Read the model definition and answer for the solid it produces. Units are mm, in the model's axes. A direction names the side the tool comes from. Coordinates: 2 decimals unless noted, no trailing zeros. Write each loop counter-clockwise with the first axis right and the second up, starting at its lowest first coordinate (ties: lowest second). Pieces come first, ordered by that corner, then holes. Notation, with made-up numbers: (18.25, 11.5) -> (36.25, 11.5) arc R23 ccw to (36.25, 43.5) -> close; hole circle Ø5 at (10, 40). An arc over 180 degrees is marked (long way). Answer as a JSON object with one key per item and string values. Group by question number.
(1) Which of the six approach directions +Z, -Z, +X, -X, +Y, -Y give full straight-line access (tool end or side, diameter ignored) to faces 4 (the face through (2.66, 200.25, -67.4)), 5 (the face through (3, 2, -12.75)), 6 (the face through (6, 175, -100)), 7 (the face through (4.93, 68.93, -91.5))?
(2) Find section A-A (y = 168.5). Give the vertices of the cut face in (x, z).
(3) Find section B-B (y = 89.4). Give the vertices of the cut face in (x, z).
(4) For a pull along Z with two mould halves and no side action, classify faces 1 (the face through (8, 8, -67)), 2 (the face through (5.4, 3, -15)), 3 (the face through (4.93, 16.93, -126.5)) as +Z half, -Z half, draft (parallel to the pull), parting line (faces both ways), or undercut.
(5) Straight lines are drawn through the part: L1, parallel to Y at x = 3.3, z = -100; L2, parallel to Z at x = 5, y = 168.5; L3, parallel to Z at x = 4.35, y = 175. For each, find the intervals that lie inside material, in ascending order.
(6) A flat-ended cylindrical pin translates along its axis: P1, Ø1.6, axis at x = 5, y = 188.5, coming from the -Z side. Find the tip coordinate at first contact, or state that the pin passes through.
from build123d import *

# Parameters (mm, degrees)
SKETCH1_W                  = 135
SKETCH1_H                  = 210
BOSS_EXTRUDE1_DEPTH        = 10
SKETCH2_W                  = 45
SKETCH2_H                  = 60
CUT_EXTRUDE1_DEPTH         = 11
SKETCH3_W                  = 10
SKETCH3_H                  = 14
SKETCH3_H_2                = 12
CUT_EXTRUDE2_DEPTH         = 11
SKETCH4_W                  = 135
SKETCH4_H                  = 10
CUT_EXTRUDE3_DEPTH         = 2
SKETCH5_R                  = 2.5
CUT_EXTRUDE4_DEPTH         = 6
CUT_EXTRUDE5_DEPTH         = 5.4
LPATTERN1_COUNT            = 3
LPATTERN1_PITCH            = 50
F_5_5_5_5_DIAMETER_HOLE1_D = 5.5
LPATTERN3_COUNT            = 3
LPATTERN3_PITCH            = 50
F_4_5_4_5_DIAMETER_HOLE1_D = 4.5
F_4_5_4_5_DIAMETER_HOLE2_D = 4.5
LPATTERN2_COUNT            = 2
LPATTERN2_PITCH            = 65
LPATTERN2_COUNT_DIR2       = 2
LPATTERN2_PITCH_DIR2       = 106
FILLET1_R                  = 5


with BuildPart() as part:
    # Sketch1 → Boss-Extrude1 (new body)
    with BuildSketch(Plane(origin=(0, 0, 0), x_dir=(0, 0, -1), z_dir=(1, 0, 0))):
        with Locations((67.5, 105)):
            Rectangle(SKETCH1_W, SKETCH1_H)
    extrude(amount=BOSS_EXTRUDE1_DEPTH)

    # Sketch2 → Cut-Extrude1 (cut, through all)
    with BuildSketch(Plane(origin=(10, 0, 0), x_dir=(0, 0, -1), z_dir=(1, 0, 0))):
        with Locations((112.5, 97.5)):
            Rectangle(SKETCH2_W, SKETCH2_H)
    extrude(amount=-CUT_EXTRUDE1_DEPTH, mode=Mode.SUBTRACT)

    # Sketch3 → Cut-Extrude2 (cut, through all)
    with BuildSketch(Plane(origin=(10, 0, 0), x_dir=(0, 0, -1), z_dir=(1, 0, 0))):
        with Locations((130, 22.5)):
            Rectangle(SKETCH3_W, SKETCH3_H)
        with Locations((130, 188.5)):
            Rectangle(SKETCH3_W, SKETCH3_H_2)
    extrude(amount=-CUT_EXTRUDE2_DEPTH, mode=Mode.SUBTRACT)

    # Sketch4 → Cut-Extrude3 (cut)
    with BuildSketch(Plane(origin=(10, 0, 0), x_dir=(0, 0, -1), z_dir=(1, 0, 0))):
        with Locations((67.5, 5)):
            Rectangle(SKETCH4_W, SKETCH4_H)
        with Locations((67.5, 205)):
            Rectangle(SKETCH4_W, SKETCH4_H)
    extrude(amount=-CUT_EXTRUDE3_DEPTH, mode=Mode.SUBTRACT)

    # Sketch5 → Cut-Extrude4 (cut)
    with BuildSketch(Plane.ZY):
        with Locations((-35, 175)):
            Circle(SKETCH5_R)
        with Locations((-100, 175)):
            Circle(SKETCH5_R)
    extrude(amount=-CUT_EXTRUDE4_DEPTH, mode=Mode.SUBTRACT)

    # Sketch6 → Cut-Extrude5 (cut)
    with BuildSketch(Plane.ZY):
        with BuildLine():
            Line((-22.25, 5), (-22.25, 0))
            Line((-22.25, 0), (-12.75, 0))
            Line((-12.75, 0), (-12.75, 5))
            ThreePointArc((-12.75, 5), (-17.5, 9.75), (-22.25, 5))
        make_face()
        with BuildLine():
            Line((-22.25, 205), (-22.25, 210))
            Line((-22.25, 210), (-12.75, 210))
            Line((-12.75, 210), (-12.75, 205))
            ThreePointArc((-12.75, 205), (-17.5, 200.25), (-22.25, 205))
        make_face()
    cut_extrude5 = extrude(amount=-CUT_EXTRUDE5_DEPTH, mode=Mode.SUBTRACT)

    # LPattern1: Cut-Extrude5 ×3
    with Locations(*[(0, 0, -i * LPATTERN1_PITCH) for i in range(1, LPATTERN1_COUNT)]):
        add(cut_extrude5, mode=Mode.SUBTRACT)

    # Ø5.5 (5.5) Diameter Hole1 (through all)
    with Locations(Plane.ZY.offset(-5.4)):
        with Locations((-17.5, 205), (-17.5, 5)):
            f_5_5_5_5_diameter_hole1 = Hole(F_5_5_5_5_DIAMETER_HOLE1_D / 2)

    # LPattern3: Ø5.5 (5.5) Diameter Hole1 ×3
    with Locations(*[(0, 0, -i * LPATTERN3_PITCH) for i in range(1, LPATTERN3_COUNT)]):
        add(f_5_5_5_5_diameter_hole1, mode=Mode.SUBTRACT)

    # Ø4.5 (4.5) Diameter Hole1 (through all)
    with Locations(Plane(origin=(10, 0, 0), x_dir=(0, 0, -1), z_dir=(1, 0, 0))):
        with Locations((15, 104.4), (50, 104.4), (15, 89.4), (50, 89.4)):
            Hole(F_4_5_4_5_DIAMETER_HOLE1_D / 2)

    # Ø4.5 (4.5) Diameter Hole2 (through all)
    with Locations(Plane(origin=(10, 0, 0), x_dir=(0, 0, -1), z_dir=(1, 0, 0))):
        with Locations((22, 36.5), (22, 62.5), (48, 62.5), (48, 36.5)):
            f_4_5_4_5_diameter_hole2 = Hole(F_4_5_4_5_DIAMETER_HOLE2_D / 2)

    # LPattern2: 4.5 _4.5_ Diameter Hole2 2 × 2
    with Locations(*[(0, j * LPATTERN2_PITCH_DIR2, -i * LPATTERN2_PITCH) for i in range(LPATTERN2_COUNT) for j in range(LPATTERN2_COUNT_DIR2) if (i, j) != (0, 0)]):
        add(f_4_5_4_5_diameter_hole2, mode=Mode.SUBTRACT)

    # Fillet1
    fillet1_edges = [part.edges().sort_by_distance(p)[0] for p in [
        (5, 67.5, -90),
        (5, 127.5, -90),
        (5, 15.5, -125),
        (5, 29.5, -125),
        (5, 182.5, -125),
        (5, 194.5, -125),
    ]]
    fillet(fillet1_edges, radius=FILLET1_R)


solid = part.part
Results below:
{
 "1": {"face 4": "-X, +Y", "face 5": "-X, -Y", "face 6": "-X", "face 7": "-Z, +X, -X"},
 "2": {"outline": "(0, -135) -> (10, -135) -> (10, -115.25) -> (0, -115.25) -> close; (0, -110.75) -> (10, -110.75) -> (10, -89.25) -> (0, -89.25) -> close; (0, -84.75) -> (10, -84.75) -> (10, -50.25) -> (0, -50.25) -> close; (0, -45.75) -> (10, -45.75) -> (10, -24.25) -> (0, -24.25) -> close; (0, -19.75) -> (10, -19.75) -> (10, 0) -> (0, 0) -> close"},
 "3": {"outline": "(0, -90) -> (10, -90) -> (10, -52.25) -> (0, -52.25) -> close; (0, -47.75) -> (10, -47.75) -> (10, -17.25) -> (0, -17.25) -> close; (0, -12.75) -> (10, -12.75) -> (10, 0) -> (0, 0) -> close"},
 "4": {"face 1": "draft", "face 2": "undercut", "face 3": "-Z half"},
 "5": {"L1": "y = 0 to 67.5, 127.5 to 172.5, 177.5 to 210", "L2": "z = -135 to -115.25, -110.75 to -89.25, -84.75 to -50.25, -45.75 to -24.25, -19.75 to 0", "L3": "z = -135 to -102.5, -97.5 to -37.5, -32.5 to 0"},
 "6": {"P1": "stops at z = -125"}
}
